Design review of the part built by this model. Coordinates are the model's own, in mm. Give positions to 0.01 mm unless a question says otherwise; leave off trailing zeros. Order: outer loops, then holes, each group sorted by start corner. A loop starts at its lowest first (then second) coordinate and runs counter-clockwise, first axis right, second up. Notation, with made-up numbers: M 39.5,10 L 58.5,10 A5 ccw 58.5,15 Z; hole C -5,89 d8. An arc over 180 degrees is marked long. Answer as a JSON object with one key per item and string values.
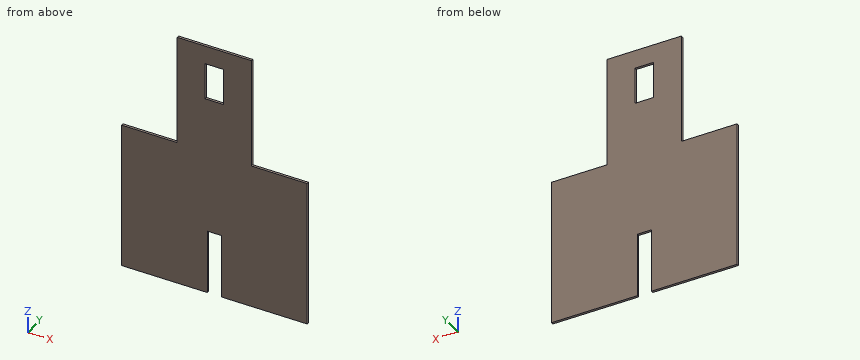
from build123d import *

# Parameters (mm, degrees)
BOSS_EXTRUDE1_DEPTH = 1.5875
CUT_EXTRUDE1_REACH  = 111.261
SKETCH2_W           = 12.7
SKETCH2_H           = 25.4
CUT_EXTRUDE2_REACH  = 111.261
SKETCH3_W           = 9.525
SKETCH3_H           = 44.45


with BuildPart() as part:
    # Sketch1 → Boss-Extrude1 (new body)
    with BuildSketch(Plane(origin=(0, 0, 0), x_dir=(1, 0, 0), z_dir=(0, 1, 0))):
        Polygon((-63.5, -12.7), (-25.4, -12.7), (-25.4, -88.9), (25.4, -88.9), (25.4, -12.7), (63.5, -12.7), (63.5, 88.9), (-63.5, 88.9), align=None)
    extrude(amount=BOSS_EXTRUDE1_DEPTH)

    # Sketch2 → Cut-Extrude1 (cut, up to next)
    with BuildSketch(Plane(origin=(0, 1.5875, 0), x_dir=(1, 0, 0), z_dir=(0, 1, 0)), mode=Mode.PRIVATE) as cut_extrude1_sk1:
        with Locations((0, -63.5)):
            Rectangle(SKETCH2_W, SKETCH2_H)
    cut_extrude1_tool1 = extrude(cut_extrude1_sk1.sketch, amount=-CUT_EXTRUDE1_REACH, mode=Mode.PRIVATE) & part.part
    add(cut_extrude1_tool1.solids().sort_by_distance((0, 1.5875, 63.5))[0], mode=Mode.SUBTRACT)

    # Sketch3 → Cut-Extrude2 (cut, up to next)
    with BuildSketch(Plane(origin=(0, 1.5875, 0), x_dir=(1, 0, 0), z_dir=(0, 1, 0)), mode=Mode.PRIVATE) as cut_extrude2_sk1:
        with Locations((0, 66.675)):
            Rectangle(SKETCH3_W, SKETCH3_H)
    cut_extrude2_tool1 = extrude(cut_extrude2_sk1.sketch, amount=-CUT_EXTRUDE2_REACH, mode=Mode.PRIVATE) & part.part
    add(cut_extrude2_tool1.solids().sort_by_distance((0, 1.5875, -66.675))[0], mode=Mode.SUBTRACT)


solid = part.part
(1) We need section B-B (y = 0.85). Write out the cut boundary in (x, z).
Checked values:
{"outline": "M -63.5,-88.9 L -4.76,-88.9 L -4.76,-44.45 L 4.76,-44.45 L 4.76,-88.9 L 63.5,-88.9 L 63.5,12.7 L 25.4,12.7 L 25.4,88.9 L -25.4,88.9 L -25.4,12.7 L -63.5,12.7 Z; hole M -6.35,50.8 L 6.35,50.8 L 6.35,76.2 L -6.35,76.2 Z"}
(2) We need section C-C (z = 60.5). Write out the cut boundary in (x, y), plus the area to 3 significant figures.
Checked values:
{"outline": "M -25.4,0 L -6.35,0 L -6.35,1.59 L -25.4,1.59 Z; M 6.35,0 L 25.4,0 L 25.4,1.59 L 6.35,1.59 Z", "area": "60.5 mm^2"}
(3) We need section D-D (x = 38.5). Write out the cut boundary in (y, z), plus the area to 3 significant figures.
Checked values:
{"outline": "M 0,-88.9 L 1.59,-88.9 L 1.59,12.7 L 0,12.7 Z", "area": "161 mm^2"}
(4) Insertion check: pin 1 (0.5 mm diameter, centred on x = 38, y = 0.5, fed in from +Z); pin 2 (0.5 mm diameter, centred on y = 1, z = 49.5, fed in from -X); pin 3 (0.8 mm diameter, centred on y = 1, z = 41.5, fed in from +X); pin 4 (12 mm diameter, centred on x = 36, z = 24, fed in from +Y). Each pin has a flat end and moves straight along its axis. Give the tip position at first contact, or say it passes through.
Checked values:
{"pin 1": "stops at z = 12.7", "pin 2": "stops at x = -25.4", "pin 3": "stops at x = 25.4", "pin 4": "passes through"}
(5) We need section A-A (z = -49.5). Write out the cut boundary in (x, y).
Checked values:
{"outline": "M -63.5,0 L -4.76,0 L -4.76,1.59 L -63.5,1.59 Z; M 4.76,0 L 63.5,0 L 63.5,1.59 L 4.76,1.59 Z"}
(6) To check wall thickness, follow L1, parallel to X at y = 0.35, z = -45.5; L2, parallel to X at y = 0.65, z = 55; L3, parallel to Z at x = 5, y = 0.9. State the ranges of each line that lie inside material, in increasing order. Write a range as from..to.
Checked values:
{"L1": "x = -63.5..-4.76, 4.76..63.5", "L2": "x = -25.4..-6.35, 6.35..25.4", "L3": "z = -88.9..50.8, 76.2..88.9"}
